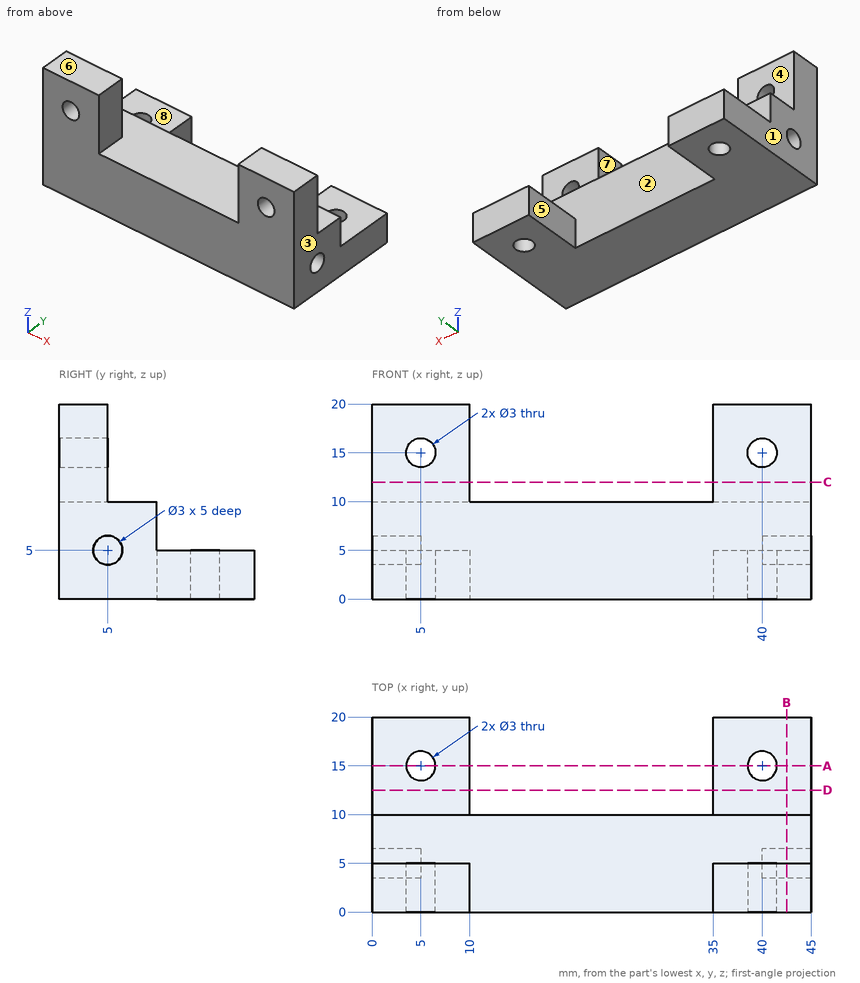
Study the drawing (mm; zero at the part's minimum x, y, z) and answer. A direction names the side the tool comes from. Round coordinates to 2 decimals unless told otherwise and drop trailing zeros. Write each loop counter-clockwise with the first axis right and the second up, starting at its lowest first coordinate (ties: lowest second). Pieces come first, ordered by that corner, then holes. Notation, with made-up numbers: (11, 47) -> (33, 47) arc R21 ccw to (33, 58) -> close; hole circle Ø1 at (75.25, 15.25). An arc over 180 degrees is marked (long way). Use CSV: the item, a comma, the result in double quotes. Start each with the question number.
(1) Section C-C on z = 12 is taken. Give the vertices of the cut face in (x, y), then the cut area to 3 significant figures.
(2) Which of the six approach directions +Z, -Z, +X, -X, +Y, -Y give full straight-line access (tool end or side, diameter ignored) to the marked faces 5, 6, 7 and 8?
(3) Section A-A on y = 15 is taken. Give the vertices of the cut face in (x, z).
(4) The mould has two halves that part along X. Classify the marked faces 1, 2, 3 and 4: released by +X, released by -X, zero draft, split by the parting line, or undercut.
(5) Section B-B on x = 42.5 is taken. Give the vertices of the cut face in (y, z).
(6) Each of these flat-tipped pins is pushed along its axis until it touches: pin 1 (2.5 mm diameter, centred on y = 5, z = 5, fed in from +X); pin 2 (3 mm diameter, centred on x = 24.5, z = 3, fed in from +Y); pin 3 (3 mm diameter, centred on x = 4.5, y = 14, fed in from +Z). Where does it stop, or does it pass through?
(7) Consider L1, parallel to Z at x = 36, y = 14.5; L2, parallel to X at y = 4.25, z = 17; L3, parallel to Z at x = 34.5, y = 3.75. Determine where each line is inside the solid, lowest interval first. Write a range as from..to.
A:
1,outline,"(0, 0) -> (10, 0) -> (10, 5) -> (0, 5) -> close; (35, 0) -> (45, 0) -> (45, 5) -> (35, 5) -> close"
1,area,"100 mm²"
2,face 5,"+Z, -Z, +Y"
2,face 6,"+Z, +X, -X, +Y, -Y"
2,face 7,"+Z, +Y, -Y"
2,face 8,"+Z, +X, -X, +Y"
3,outline,"(0, 0) -> (3.5, 0) -> (3.5, 5) -> (0, 5) -> close; (6.5, 0) -> (10, 0) -> (10, 5) -> (6.5, 5) -> close; (35, 0) -> (38.5, 0) -> (38.5, 5) -> (35, 5) -> close; (41.5, 0) -> (45, 0) -> (45, 5) -> (41.5, 5) -> close"
4,face 1,"released by -X"
4,face 2,"undercut"
4,face 3,"released by +X"
4,face 4,"zero draft"
5,outline,"(0, 0) -> (20, 0) -> (20, 5) -> (10, 5) -> (10, 10) -> (5, 10) -> (5, 20) -> (0, 20) -> close; hole circle Ø3 at (5, 5)"
6,pin 1,"stops at x = 40"
6,pin 2,"stops at y = 10"
6,pin 3,"stops at z = 5"
7,L1,"z = 0..5"
7,L2,"x = 0..10, 35..45"
7,L3,"z = 0..10"
